from build123d import *

# Parameters (mm, degrees)
F0_R     = 12.7
F1_DEPTH = 3.175
F2_R     = 4.7625
F3_DEPTH = 17.4625
F4_DEPTH = 25.4


# Not quite as in the source:
# - a length typed as a fraction of an inch, garbled in the dataset ("3 / 203.2 mm" for 3/8 in), is restored


with BuildPart() as f1:
    # F0 (on Top) → F1 (new body)
    with BuildSketch(Plane.XY):
        Circle(F0_R)
        with BuildLine():
            ThreePointArc((2.1403987868, 2.67081), (0, -3.42265), (-2.1403987868, 2.67081))
            Line((-2.1403987868, 2.67081), (2.1403987868, 2.67081))
        make_face(mode=Mode.SUBTRACT)
    extrude(amount=F1_DEPTH)

    # F2 (on face) → F3 (join)
    with BuildSketch(Plane.XY.offset(3.175)):
        Circle(F2_R)
        with BuildLine():
            Line((-2.1403987868, 2.67081), (2.1403987868, 2.67081))
            ThreePointArc((2.1403987868, 2.67081), (0, -3.42265), (-2.1403987868, 2.67081))
        make_face(mode=Mode.SUBTRACT)
    extrude(amount=F3_DEPTH)

    # F2 (on face) → F4 (cut)
    with BuildSketch(Plane.XY.offset(3.175)):
        with BuildLine():
            ThreePointArc((-4.8118133156, 7.58825), (-3.6688133156, 8.73125), (-4.8118133156, 9.87425))
            Line((-4.8118133156, 9.87425), (-7.9868133156, 9.87425))
            ThreePointArc((-7.9868133156, 9.87425), (-9.1568912319, 8.8000763046), (-10.1837351663, 7.58825))
            Line((-10.1837351663, 7.58825), (-4.8118133156, 7.58825))
        make_face()
    extrude(amount=-F4_DEPTH, mode=Mode.SUBTRACT)


solid = f1.part
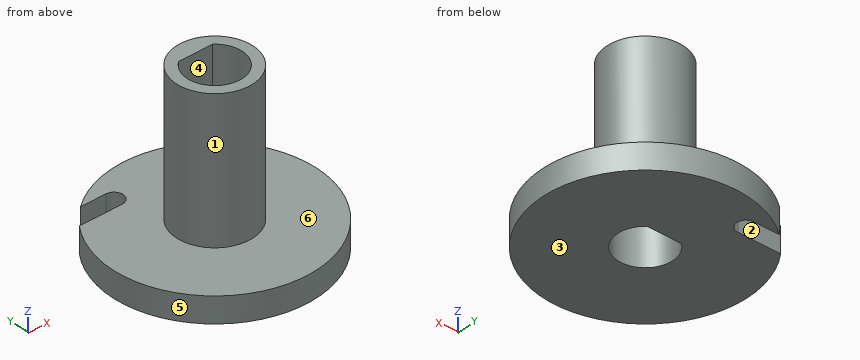
Check sheet for the modelled part. Datum: model origin and axes. Units: mm. Face numbers are marked on the shaded views. A direction names the side the tool comes from. Round coordinates to 2 decimals unless told otherwise and drop trailing zeros. Loops run counter-clockwise (first coordinate to the right, second up) from the corner with the lowest first, then second, coordinate; pieces in that order, holes last. Notation, with made-up numbers: (66.25, 53.25) -> (74.25, 53.25) arc R13 ccw to (74.25, 73.25) -> close; hole circle Ø2 at (69.25, 78.25). An arc over 180 degrees is marked (long way). Put each result on its own line as item: value. Start each with the question number.
1. Scan lines: probe 1 along Y at (x, z) = (0, 9.5); probe 2 along X at (y, z) = (-2.5, 9.25); probe 3 along Z at (x, y) = (-9, 5.25) (3 decimals). Record each from-to range of solid material in increasing order.
2. Section check A-A (x = 0). Enter the section's corners in (y, z) (1 decimal), plus the area to 3 significant figures.
3. Access from +Z, -Z, +X, -X, +Y, -Y to the whole of each face (thin tool, end or side, straight path). Record for the marked faces 1, 2 and 3.
4. Draft check along X on the marked faces 4, 5 and 6. Enter one of: +X half, -X half, draft (parallel to the pull), parting line (faces both ways), or undercut.
5. Section check D-D (z = 18.5). Enter the section's corners in (x, y) (1 decimal), plus the area to 3 significant figures.
6. Section check B-B (y = 0). Enter the section's corners in (x, z) (1 decimal).
7. Gauge pin test, flat ends, axial feed: pin 1 (10 mm diameter, centred on x = 9.5, y = 9, fed in from -Z); pin 2 (2 mm diameter, centred on x = -2.5, z = 13.5, fed in from -Y); pin 3 (1 mm diameter, centred on x = -7.5, z = 1.5, fed in from +Y); pin 4 (8 mm diameter, centred on x = 6, z = 2.5, fed in from +Y). Record the tip position at first contact, or that the pin passes through.
8. Section check C-C (z = 2). Enter the section's corners in (x, y), plus the area to 3 significant figures.
Findings:
1. probe 1: y = -4.76 to -3.42, 2.67 to 4.76
1. probe 2: x = -4.05 to -2.34, 2.34 to 4.05
1. probe 3: z = 0 to 3.175
2. outline: (-12.7, 0) -> (-3.4, 0) -> (-3.4, 20.6) -> (-4.8, 20.6) -> (-4.8, 3.2) -> (-12.7, 3.2) -> close; (2.7, 0) -> (12.7, 0) -> (12.7, 3.2) -> (4.8, 3.2) -> (4.8, 20.6) -> (2.7, 20.6) -> close
2. area: 121 mm^2
3. face 1: +Z
3. face 2: +Z, -Z, -X
3. face 3: -Z, +X, -X, +Y, -Y
4. face 4: undercut
4. face 5: parting line
4. face 6: draft
5. outline: circle Ø9.5 at (0, 0); hole (-2.1, 2.7) arc R3.4 ccw (long way) to (2.1, 2.7) -> close
5. area: 36.7 mm^2
6. outline: (-12.7, 0) -> (-3.4, 0) -> (-3.4, 20.6) -> (-4.8, 20.6) -> (-4.8, 3.2) -> (-12.7, 3.2) -> close; (3.4, 0) -> (12.7, 0) -> (12.7, 3.2) -> (4.8, 3.2) -> (4.8, 20.6) -> (3.4, 20.6) -> close
7. pin 1: stops at z = 0
7. pin 2: stops at y = -4.52
7. pin 3: stops at y = 10.6
7. pin 4: stops at y = 12.54
8. outline: (-10.18, 7.59) arc R12.7 ccw (long way) to (-7.99, 9.87) -> (-4.81, 9.87) arc R1.14 cw to (-4.81, 7.59) -> close; hole (-2.14, 2.67) arc R3.42 ccw (long way) to (2.14, 2.67) -> close
8. area: 460 mm^2
